Here's the drawing with two shaded views (mm, measured from the low corner). I have some questions. Coordinates: 2 decimals unless noted, no trailing zeros. Loops run counter-clockwise (first coordinate to the right, second up) from the corner with the lowest first, then second, coordinate; pieces in that order, holes last. Notation, with made-up numbers: (-32.75, 23.25) - (-19.75, 23.25) arc R28 ccw to (-19.75, 58.25) - close; hole circle Ø3 at (84, -34.5). An arc over 180 degrees is marked (long way). Use a Markdown table: item, result.
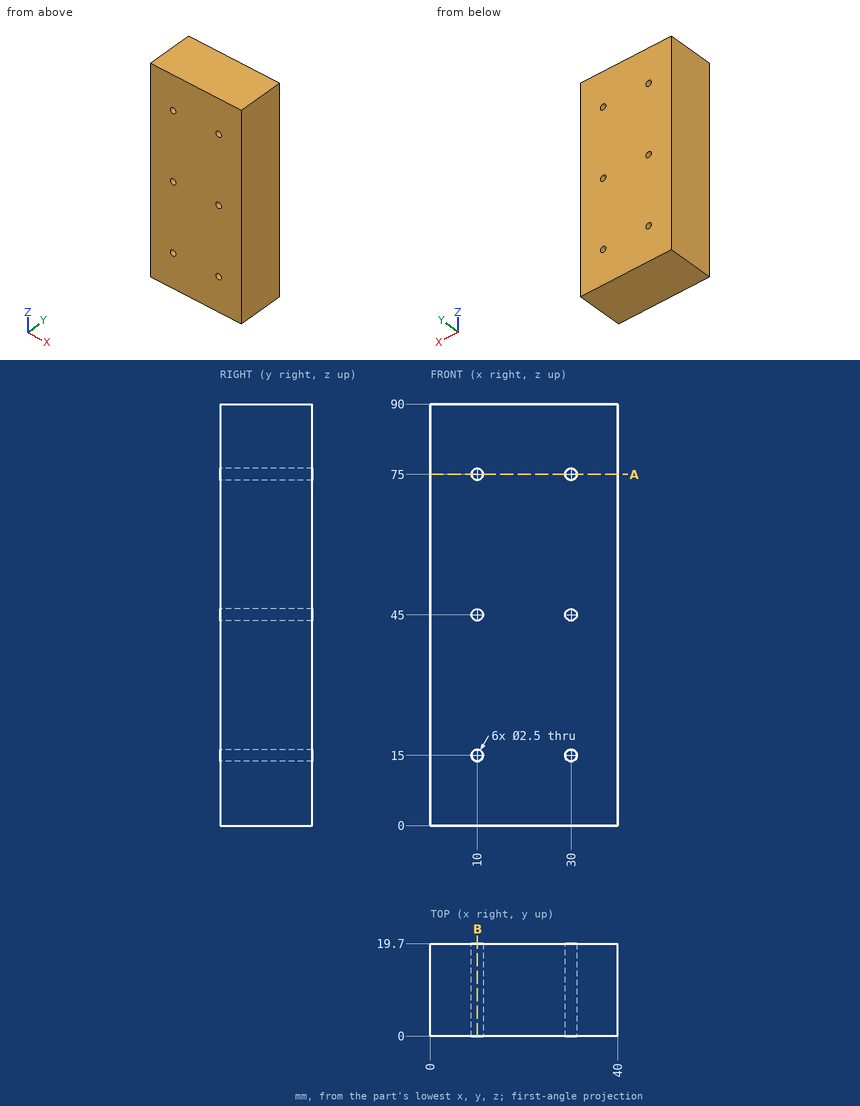
Q1. Please list where these lines run through material, in increasing order: L1, parallel to Z at x = 30, y = 10.5; L2, parallel to X at y = 4.5, z = 75; L3, parallel to Z at x = 29, y = 5.5. Write a range as from..to.
Check values:
| item | result |
|---|---|
| L1 | 0..13.75, 16.25..43.75, 46.25..73.75, 76.25..90 |
| L2 | 0..8.75, 11.25..28.75, 31.25..40 |
| L3 | 0..14.25, 15.75..44.25, 45.75..74.25, 75.75..90 |
Q2. I want a section at A-A, the plane z = 75. Write out the boundary of the cut face in (x, y), then the cut area to 4 significant figures.
Check values:
| item | result |
|---|---|
| outline | (0, 0) - (8.75, 0) - (8.75, 19.7) - (0, 19.7) - close; (11.25, 0) - (28.75, 0) - (28.75, 19.7) - (11.25, 19.7) - close; (31.25, 0) - (40, 0) - (40, 19.7) - (31.25, 19.7) - close |
| area | 689.5 mm^2 |
Q3. Will this pin go through, and if not, where does the flat tip stop? P1, Ø2, axis at x = 10, z = 75, coming from the +Y side.
Check values:
| item | result |
|---|---|
| P1 | through |
Q4. I want a section at B-B, the plane x = 10. Write out the boundary of the cut face in (y, z).
Check values:
| item | result |
|---|---|
| outline | (0, 0) - (19.7, 0) - (19.7, 13.75) - (0, 13.75) - close; (0, 16.25) - (19.7, 16.25) - (19.7, 43.75) - (0, 43.75) - close; (0, 46.25) - (19.7, 46.25) - (19.7, 73.75) - (0, 73.75) - close; (0, 76.25) - (19.7, 76.25) - (19.7, 90) - (0, 90) - close |
